from build123d import *

# Parameters (mm, degrees)
EXTRUDE_1_DEPTH     = 3
EXTRUDE_1_2_DEPTH   = 2
SKETCH_3_R          = 1.3
CUT_EXTRUDE_1_DEPTH = 5
CHAMFER_1_SIZE      = 3


with BuildPart() as part:
    # Эскиз1 → Extrude 1 (new body)
    with BuildSketch(Plane.XY):
        with BuildLine():
            Line((-64.25, 60.75), (-64.25, -60.75))
            ThreePointArc((-64.25, -60.75), (-63.371320344, -62.871320344), (-61.25, -63.75))
            Line((-61.25, -63.75), (61.25, -63.75))
            ThreePointArc((61.25, -63.75), (63.371320344, -62.871320344), (64.25, -60.75))
            Line((64.25, -60.75), (64.25, 60.75))
            ThreePointArc((64.25, 60.75), (63.371320344, 62.871320344), (61.25, 63.75))
            Line((61.25, 63.75), (-61.25, 63.75))
            ThreePointArc((-61.25, 63.75), (-63.371320344, 62.871320344), (-64.25, 60.75))
        make_face()
    extrude(amount=EXTRUDE_1_DEPTH)

    # Эскиз2 → Extrude 1 2 (add)
    with BuildSketch(Plane(origin=(0, 0, 0), x_dir=(-1, 0, 0), z_dir=(0, 0, -1))):
        with BuildLine():
            Line((-44.25, -57.75), (44.25, -57.75))
            ThreePointArc((44.25, -57.75), (47.078427125, -56.578427125), (48.25, -53.75))
            ThreePointArc((48.25, -53.75), (50.007359313, -49.507359313), (54.25, -47.75))
            ThreePointArc((54.25, -47.75), (57.078427125, -46.578427125), (58.25, -43.75))
            Line((58.25, -43.75), (58.25, 43.75))
            ThreePointArc((58.25, 43.75), (57.078427125, 46.578427125), (54.25, 47.75))
            ThreePointArc((54.25, 47.75), (50.007359313, 49.507359313), (48.25, 53.75))
            ThreePointArc((48.25, 53.75), (47.078427125, 56.578427125), (44.25, 57.75))
            Line((44.25, 57.75), (-44.25, 57.75))
            ThreePointArc((-44.25, 57.75), (-47.078427125, 56.578427125), (-48.25, 53.75))
            ThreePointArc((-48.25, 53.75), (-50.007359313, 49.507359313), (-54.25, 47.75))
            ThreePointArc((-54.25, 47.75), (-57.078427125, 46.578427125), (-58.25, 43.75))
            Line((-58.25, 43.75), (-58.25, -43.75))
            ThreePointArc((-58.25, -43.75), (-57.078427125, -46.578427125), (-54.25, -47.75))
            ThreePointArc((-54.25, -47.75), (-50.007359313, -49.507359313), (-48.25, -53.75))
            ThreePointArc((-48.25, -53.75), (-47.078427125, -56.578427125), (-44.25, -57.75))
        make_face()
        with BuildLine():
            Line((-44.25, -54.75), (44.25, -54.75))
            ThreePointArc((44.25, -54.75), (44.957106781, -54.457106781), (45.25, -53.75))
            ThreePointArc((45.25, -53.75), (47.886038969, -47.386038969), (54.25, -44.75))
            ThreePointArc((54.25, -44.75), (54.957106781, -44.457106781), (55.25, -43.75))
            Line((55.25, -43.75), (55.25, 43.75))
            ThreePointArc((55.25, 43.75), (54.957106781, 44.457106781), (54.25, 44.75))
            ThreePointArc((54.25, 44.75), (47.886038969, 47.386038969), (45.25, 53.75))
            ThreePointArc((45.25, 53.75), (44.957106781, 54.457106781), (44.25, 54.75))
            Line((44.25, 54.75), (-44.25, 54.75))
            ThreePointArc((-44.25, 54.75), (-44.957106781, 54.457106781), (-45.25, 53.75))
            ThreePointArc((-45.25, 53.75), (-47.886038969, 47.386038969), (-54.25, 44.75))
            ThreePointArc((-54.25, 44.75), (-54.957106781, 44.457106781), (-55.25, 43.75))
            Line((-55.25, 43.75), (-55.25, -43.75))
            ThreePointArc((-55.25, -43.75), (-54.957106781, -44.457106781), (-54.25, -44.75))
            ThreePointArc((-54.25, -44.75), (-47.886038969, -47.386038969), (-45.25, -53.75))
            ThreePointArc((-45.25, -53.75), (-44.957106781, -54.457106781), (-44.25, -54.75))
        make_face(mode=Mode.SUBTRACT)
    extrude(amount=EXTRUDE_1_2_DEPTH)

    # Эскиз3 → Вырез-Вытянуть1 (cut)
    with BuildSketch(Plane.XY.offset(3)):
        with Locations((54.25, -53.75)):
            Circle(SKETCH_3_R)
        with Locations((54.25, 53.75)):
            Circle(SKETCH_3_R)
        with Locations((-54.25, 53.75)):
            Circle(SKETCH_3_R)
        with Locations((-54.25, -53.75)):
            Circle(SKETCH_3_R)
    extrude(amount=-CUT_EXTRUDE_1_DEPTH, mode=Mode.SUBTRACT)

    # Фаска1
    chamfer_1_edges = [part.edges().sort_by_distance(p)[0] for p in [
        (-55.55, -53.75, 3),
        (-55.55, 53.75, 3),
        (52.95, 53.75, 3),
        (52.95, -53.75, 3),
    ]]
    chamfer(chamfer_1_edges, length=CHAMFER_1_SIZE - 0.0001)  # a hair under: the kernel refuses the full size


solid = part.part
Source: CAD feature listing. Evaluate the final solid. Frame: model axes, mm. A direction names the side the tool comes from. Round coordinates to 2 decimals unless told otherwise and drop trailing zeros. Order: outer loops, then holes, each group sorted by start corner. A loop starts at its lowest first (then second) coordinate and runs counter-clockwise, first axis right, second up. Notation, with made-up numbers: (-39.75, 66.5) - (-18.75, 66.5) arc R18 cw to (-18.75, 100.5) - close; hole circle Ø6 at (37, -9). An arc over 180 degrees is marked (long way). Use a Markdown table: item, result. Add a question column.
1. Mould query, pull axis X, two halves, no side actions, for faces 4 (the flat face through (-64.25, 1, 1)), 5 (the flat face through (-1, -63.75, 1)), 6 (the flat face through (-1, 1, 0)). Classes: +X half, -X half, draft (parallel to the pull), parting line (faces both ways), or undercut.
2. Section query A-A (y = 19). Return the cut outline in (x, z).
3. First-contact query: pin 1 (4 mm diameter, centred on x = 54.25, y = 53.75, fed in from -Z); pin 2 (0.6 mm diameter, centred on y = 17, z = -1, fed in from +X); pin 3 (1.6 mm diameter, centred on x = -9, z = -1.5, fed in from -Y); pin 4 (2 mm diameter, centred on x = 54.25, y = -53.75, fed in from -Z). Flat tips, straight axial feed; report the tip coordinate or a pass-through.
4. Line query: probe 1 along Y at (x, z) = (-3.5, -1.2); probe 2 along X at (y, z) = (53.75, 0.05); probe 3 along Y at (x, z) = (52, 2.3). Output: solid intervals per line, ascending.
5. Section query B-B (x = -11.5). Return the cut outline in (y, z).
6. Set-up query: faces 1 (the cylindrical face through (49.961, 49.554, -0.986)), 2 (the cylindrical face through (47.816, 47.456, -0.986)), 3 (the cylindrical face through (-57.109, 46.547, -0.986)). Return all of +Z, -Z, +X, -X, +Y, -Y with unobstructed straight access to the full face (end or side cutting, diameter ignored); none if empty.
Derived:
| question | item | result |
|---|---|---|
| 1 | face 4 | -X half |
| 1 | face 5 | draft |
| 1 | face 6 | undercut |
| 2 | outline | (-64.25, 0) - (-58.25, 0) - (-58.25, -2) - (-55.25, -2) - (-55.25, 0) - (55.25, 0) - (55.25, -2) - (58.25, -2) - (58.25, 0) - (64.25, 0) - (64.25, 3) - (-64.25, 3) - close |
| 3 | pin 1 | z = 0 |
| 3 | pin 2 | x = 58.25 |
| 3 | pin 3 | y = -57.75 |
| 3 | pin 4 | through |
| 4 | probe 1 | -57.75 to -54.75, 54.75 to 57.75 |
| 4 | probe 2 | -64.25 to -55.6, -52.9 to 52.9, 55.6 to 64.25 |
| 4 | probe 3 | -63.75 to -56.56, -50.94 to 50.94, 56.56 to 63.75 |
| 5 | outline | (-63.75, 0) - (-57.75, 0) - (-57.75, -2) - (-54.75, -2) - (-54.75, 0) - (54.75, 0) - (54.75, -2) - (57.75, -2) - (57.75, 0) - (63.75, 0) - (63.75, 3) - (-63.75, 3) - close |
| 6 | face 1 | -Z, +X, +Y |
| 6 | face 2 | -Z |
| 6 | face 3 | -Z, -X, +Y |
